Read the model definition and answer for the solid it produces. Units are mm, in the model's axes. Face numbers are marked on the shaded views. A direction names the side the tool comes from. Coordinates: 2 decimals unless noted, no trailing zeros. Write each loop counter-clockwise with the first axis right and the second up, starting at its lowest first coordinate (ties: lowest second). Pieces come first, ordered by that corner, then holes. Notation, with made-up numbers: M -10,22.5 L 3,22.5 A33 cw 3,52.5 Z; hole C 25,10 d2. An arc over 180 degrees is marked long. Write item = value, one per line.
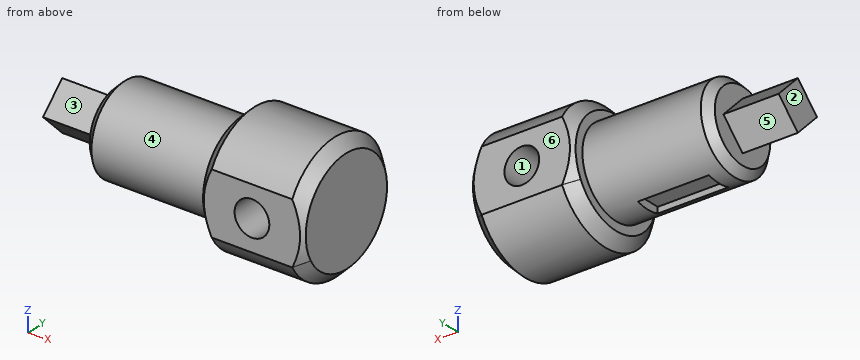
from build123d import *

# Parameters (mm, degrees)
EXTRUDE_1_DEPTH          = 35
SKETCH_4_W               = 45.00000000000001
SKETCH_4_H               = 5
CUT_EXTRUDE_1_DEPTH      = 8
CUT_EXTRUDE_2_DEPTH      = 189.67962264113208
CUT_EXTRUDE_3_DEPTH      = 166.90660023037057
CUT_EXTRUDE_3_DEPTH_BACK = 166.90660023037057
SKETCH_6_R               = 10.999999999999993
CHAMFER_1_SIZE           = 7
CHAMFER_2_SIZE           = 5


with BuildPart() as part:
    # Эскиз1 → Повернуть1 (revolve)
    with BuildSketch(Plane.XY, mode=Mode.PRIVATE) as revolve_1_sk:
        Polygon((0, 0), (0, 27.5), (80, 27.500000000000004), (80, 40.00000000000001), (145, 40.00000000000001), (145, 1e-17), align=None)
    revolve(revolve_1_sk.sketch.rotate(Axis((0, 0, 0), (-1, 0, 0)), 90), axis=Axis((0, 0, 0), (-1, 0, 0)))

    # Эскиз3 → Бобышка-Вытянуть1 (add)
    with BuildSketch(Plane.ZY):
        Polygon((-1.63e-15, -15.556349186104034), (-15.556349186104049, 8.31e-15), (-6.49e-15, 15.55634918610405), (15.55634918610404, 8.54e-15), align=None)
    extrude(amount=EXTRUDE_1_DEPTH)

    # Эскиз4 → Вырез-Вытянуть1 (cut, symmetric)
    with BuildSketch(Plane(origin=(0, 0, 0), x_dir=(1, 0, 0), z_dir=(0, 1, 0))):
        with Locations((37.50000000000001, 25.000000000000004)):
            Rectangle(SKETCH_4_W, SKETCH_4_H)
    extrude(amount=CUT_EXTRUDE_1_DEPTH, both=True, mode=Mode.SUBTRACT)

    # Эскиз5 → Вырез-Вытянуть2 (cut, symmetric)
    with BuildSketch(Plane(origin=(145, 0, 0), x_dir=(0, 0, -1), z_dir=(1, 0, 0))):
        Polygon((-220.66774826766613, 35), (-19.364916731037095, 35), (19.364916731037095, 35), (220.66774826766613, 35), (220.66774826766613, 437.6056630732581), (-220.66774826766613, 437.6056630732581), align=None)
    cut_extrude_2 = extrude(amount=CUT_EXTRUDE_2_DEPTH, both=True, mode=Mode.SUBTRACT)

    # Зеркальное отражение1: Вырез-Вытянуть2 across plane
    add(cut_extrude_2.mirror(Plane.ZX), mode=Mode.SUBTRACT)

    # Эскиз6 → Вырез-Вытянуть3 (cut, two sides: drawn at the far end of the back side and taken through both)
    with BuildSketch(Plane(origin=(0, 35, 0), x_dir=(1, 0, 0), z_dir=(0, 1, 0)).offset(-CUT_EXTRUDE_3_DEPTH_BACK)):
        with Locations(Location((112.5, 0, 0), (0, 0, 270))):
            Circle(SKETCH_6_R)
    extrude(amount=CUT_EXTRUDE_3_DEPTH + CUT_EXTRUDE_3_DEPTH_BACK, mode=Mode.SUBTRACT)

    # Фаска1
    chamfer_1_edges = [part.edges().sort_by_distance(p)[0] for p in [
        (80, 3.55e-15, -40.00000000000001),
    ]]
    chamfer(chamfer_1_edges, length=CHAMFER_1_SIZE)
    chamfer_1_2_edges = [part.edges().sort_by_distance(p)[0] for p in [
        (80, -1.421e-14, 40.000000000000014),
    ]]
    chamfer(chamfer_1_2_edges, length=CHAMFER_1_SIZE - 0.0001)  # a hair under: the kernel refuses the full size
    chamfer_1_3_edges = [part.edges().sort_by_distance(p)[0] for p in [
        (145, 3.55e-15, -40.00000000000001),
    ]]
    chamfer(chamfer_1_3_edges, length=CHAMFER_1_SIZE)
    chamfer_1_4_edges = [part.edges().sort_by_distance(p)[0] for p in [
        (145, -1.421e-14, 40.000000000000014),
    ]]
    chamfer(chamfer_1_4_edges, length=CHAMFER_1_SIZE - 0.0001)  # a hair under: the kernel refuses the full size

    # Фаска2
    chamfer_2_edges = [part.edges().sort_by_distance(p)[0] for p in [
        (0, -6.42e-15, 27.5),
    ]]
    chamfer(chamfer_2_edges, length=CHAMFER_2_SIZE)


solid = part.part
Item 1: Find section A-A (x = 112.5). Determine the outline of the cut face in (y, z), and give its area (3 significant figures).
Worked answers:
outline = M -35,-19.36 A40 ccw 35,-19.36 L 35,-11 L -35,-11 Z; M -35,11 L 35,11 L 35,19.36 A40 ccw -35,19.36 Z
area = 3,220 mm²
Item 2: For a pull along X with two mould halves and no side action, classify the marked faces 1, 2 and 3 as released by +X, released by -X, zero draft, split by the parting line, or undercut.
Worked answers:
face_1 = undercut
face_2 = released by -X
face_3 = zero draft
Item 3: Find section B-B (x = 50). Determine the outline of the cut face in (y, z), and give its area (3 significant figures).
Worked answers:
outline = M -8,-26.31 L -8,-22.5 L 8,-22.5 L 8,-26.31 A27.5 ccw long Z
area = 2,300 mm²
Item 4: Which of the six approach directions +Z, -Z, +X, -X, +Y, -Y give full straight-line access (tool end or side, diameter ignored) to the marked faces 4, 5 and 6?
Worked answers:
face_4 = -X
face_5 = -Z, -X, +Y
face_6 = +Z, -Z, +X, -X, +Y
Item 5: Flat-ended cylindrical pins translate along their axes: pin 1 (2.5 mm diameter, centred on y = -3.5, z = -24, fed in from -X); pin 2 (1.1 mm diameter, centred on x = 48, z = -24.5, fed in from -Y); pin 3 (4 mm diameter, centred on x = 86, y = 27, fed in from -Z). Find the tip coordinate at first contact, or state that the pin passes through.
Worked answers:
pin_1 = 0.5
pin_2 = -13.51
pin_3 = -31.01
Item 6: Consider line 1 along X through (y, z) = (17, 0); line 2 along X through (y, z) = (7.5, 0); line 3 along Z through (x, y) = (112.5, -12.5). Determine where each line is inside the solid, lowest interval first. Write a range as from..to.
Worked answers:
line_1 = 0..101.5, 123.5..145
line_2 = -35..101.5, 123.5..145
line_3 = -38..-11, 11..38
